Model file for the job. Use its own axes, mm. Face numbers are marked on the shaded views. Give positions to 0.01 mm unless a question says otherwise; leave off trailing zeros. Write each loop counter-clockwise with the first axis right and the second up, starting at its lowest first coordinate (ties: lowest second). Pieces come first, ordered by that corner, then holes. Notation, with made-up numbers: (71, 54) - (110, 54) arc R22 cw to (110, 63) - close; hole circle Ø7 at (18, 51). An arc over 180 degrees is marked (long way). One line per item, written item: value. Start each with the question number.
(1) Cut at C-C, the plane y = -13. List the corners of the cut face in (x, z).
(2) Probe L1, parallel to Y at x = 52.5, z = -2.5; L2, parallel to Y at x = 27, z = 11.25; L3, parallel to Y at x = 23, z = 8. List the from-to ranges inside material, lowest first.
(3) Cut at A-A, the plane z = -2.25. List the corners of the cut face in (x, y), and give its area (3 significant figures).
(4) Mould opens along X. For the marked faces 1, 2 and 3 say: pulls with the +X half, pulls with the -X half, needs draft (parallel to the pull), parting line crosses it, or undercut.
(5) Cut at D-D, the plane z = 10. State how many separate pieces and enclosed holes the cut face has, and give its area (3 significant figures).
(6) Drop flat-ended pins along their axis: P1, Ø10, axis at y = 12.5, z = 4.5, coming from the +X side; P2, Ø4.5, axis at x = 22.5, z = 9.5, coming from the -Y side; P3, Ø1, axis at y = 22, z = 3.5, coming from the -X side. Give the stop position or say it passes through.
(7) Cut at B-B, the plane y = 4. List the corners of the cut face in (x, z).
Autodesk Fusion 360 part; units mm, degrees
sketch "Sketch5" plane through (0, 0, 0) normal (1, 0, 0) x (0, 1, 0)
  line L0 (-20, 0) -> (20, 0)
  arc A0 (20, 0) -> (-20, 0) centre (0, -65.1667) ccw
  line L1 (-9.145, 3) -> (16.9339, 3) construction
  line L2 (-20, 0) -> (20, 0)
  line L3 (20, 0) -> (20, -3)
  line L4 (20, -3) -> (-20, -3)
  line L5 (-20, -3) -> (-20, 0)
  dimension "d18" = 3
  dimension "d19" = 40
  dimension "d20" = 3
extrude "Extrude5" add sketch "Sketch5" along normal blind 70 makes body 1
sketch "Sketch6" plane through (0, 0, -3) normal (0, 0, -1) x (1, 0, 0)
  line L0 (0, 20) -> (0, -20)
  line L1 (0, -20) -> (70, -20)
  line L2 (70, -20) -> (70, 20)
  line L3 (70, 20) -> (0, 20)
  line L4 (32.5, -5) -> (47.5, -5)
  arc A0 (47.5, -5) -> (47.5, 5) centre (47.5, 0) ccw
  line L5 (47.5, 5) -> (32.5, 5)
  arc A1 (32.5, 5) -> (32.5, -5) centre (32.5, 0) ccw
  line L6 (32.5, 0) -> (47.5, 0) construction
  line L7 (0, 0) -> (70, 0) construction
  line L8 (40, 5) -> (40, -5) construction
  dimension "d23" = 10
  dimension "d24" = 15
  dimension "d25" = 40
extrude "Extrude6" cut sketch "Sketch6" against normal through all contours L4 A0 L5 A1 bodies 1
ref_plane "WorkPlane3" through (0, 12.125, 0) normal (-0.9659, 0, 0.2588) x (0, 1, 0)
sketch "Sketch7" plane through (0, 12.125, 0) normal (-0.9659, 0, 0.2588) x (0, 1, 0)
  line L0 (10.375, 0) -> (-34.625, 0)
  line L1 (-34.625, 0) -> (-34.625, -25)
  line L2 (-34.625, -25) -> (10.375, -25)
  line L3 (10.375, -25) -> (10.375, 0)
  line L4 (-10.375, 0) -> (10.375, 0)
  point P0 (-12.125, 0)
  dimension "d28" = 45
  dimension "d29" = 25
extrude "Extrude7" add sketch "Sketch7" along normal blind 45 bodies 1
extrude "Extrude8" add 1 faces at (-28.9778, -6.6667, 7.7646) along direction (-0.258819, 0, -0.965926) blind 55 on bodies 1 bodies 1
ref_plane "WorkPlane4" through (16.4027, 0, 3) normal (0, 0, 1) x (0, 1, 0)
sketch "Sketch8" plane through (16.4027, 0, 3) normal (0, 0, 1) x (1, 0, 0)
  line L0 (16.0973, 5) -> (31.0973, 5)
  spline S0 degree 3 poles (31.0973, 5) (31.7254, 5) (32.3951, 4.8744) (33.627, 4.3641) (34.189, 3.9793) (35.0767, 3.0917) (35.4614, 2.5296) (35.9718, 1.2978) (36.0973, 0.6281) (36.0973, -0.6281) (35.9718, -1.2978) (35.4614, -2.5296) (35.0767, -3.0917) (34.189, -3.9793) (33.627, -4.3641) (32.3951, -4.8744) (31.7254, -5) (31.0973, -5) knots -1.507328 -1.507328 -1.507328 -1.507328 -1.318912 -1.318912 -1.130496 -1.130496 -0.94208 -0.94208 -0.753664 -0.753664 -0.565248 -0.565248 -0.376832 -0.376832 -0.188416 -0.188416 0 0 0 0
  line L1 (31.0973, -5) -> (16.0973, -5)
  spline S1 degree 3 poles (16.0973, -5) (15.4693, -5) (14.7995, -4.8744) (13.5677, -4.3641) (13.0056, -3.9793) (12.118, -3.0917) (11.7332, -2.5296) (11.2229, -1.2978) (11.0973, -0.6281) (11.0973, 0.6281) (11.2229, 1.2978) (11.7332, 2.5296) (12.118, 3.0917) (13.0056, 3.9793) (13.5677, 4.3641) (14.7995, 4.8744) (15.4693, 5) (16.0973, 5) knots 0 0 0 0 0.188416 0.188416 0.376832 0.376832 0.565248 0.565248 0.753664 0.753664 0.94208 0.94208 1.130496 1.130496 1.318912 1.318912 1.507328 1.507328 1.507328 1.507328
  line L2 (23.5973, 5) -> (23.5973, -5) construction
  circle A0 centre (23.5973, 0) radius 16
  circle A1 centre (23.5973, 0) radius 13
  dimension "d35" = 32
  dimension "d36" = 26
ref_plane "WorkPlane5" through (40, 0, 3) normal (0.2588, 0, 0.9659) x (0, -1, 0)
ref_plane "WorkPlane6" through (42.0706, 0, 10.7274) normal (0.2588, 0, 0.9659) x (0, -1, 0)
sketch "Sketch10" plane through (42.0706, 0, 10.7274) normal (0.2588, 0, 0.9659) x (0, -1, 0)
  line L0 (21, -21) -> (-21, 21) construction
  line L1 (21, -21) -> (-21, -21)
  line L2 (-21, -21) -> (-21, 21)
  line L3 (-21, 21) -> (21, 21)
  line L4 (21, 21) -> (21, -21)
  line L5 (21, -17) -> (17, -21)
  line L6 (-17, -21) -> (-21, -17)
  line L7 (-21, 17) -> (-17, 21)
  line L8 (21, 17) -> (17, 21)
  line L9 (-21, -17) -> (-23, -17)
  line L10 (-23, -17) -> (-23, 17)
  line L11 (-23, 17) -> (-21, 17)
  line L12 (-21, 17) -> (-21, -17)
  line L13 (21, -17) -> (23, -17)
  line L14 (23, -17) -> (23, 17)
  line L15 (23, 17) -> (21, 17)
  line L16 (21, 17) -> (21, -17)
  circle A0 centre (0, 0) radius 11.5
  line L17 (15.5, -15.5) -> (-15.5, -15.5) construction
  line L18 (-15.5, -15.5) -> (-15.5, 15.5) construction
  line L19 (-15.5, 15.5) -> (15.5, 15.5) construction
  line L20 (15.5, 15.5) -> (15.5, -15.5) construction
  line L21 (0, -21) -> (0, -15.5) construction
  line L22 (0, 15.5) -> (0, 21) construction
  circle A1 centre (15.5, -15.5) radius 1.75
  circle A2 centre (-15.5, -15.5) radius 1.75
  circle A3 centre (15.5, 15.5) radius 1.75
  circle A4 centre (-15.5, 15.5) radius 1.75
  circle A5 centre (15.5, -15.5) radius 3.25
  circle A6 centre (-15.5, -15.5) radius 3.25
  circle A7 centre (-15.5, 15.5) radius 3.25
  circle A8 centre (15.5, 15.5) radius 3.25
  dimension "d64" = 42
  dimension "d65" = 4
  dimension "d66" = 2
  dimension "d67" = 2
  dimension "d75" = 23
  dimension "d76" = 31
  dimension "d77" = 3.5
  dimension "d78" = 6.5
extrude "Extrude16" add sketch "Sketch10" along normal up to surface from surface at 2 separate body contours L1 L2 L3 L4 L5 L6 L7 L8 L12 L16 | A5 | A6 | A7 | A8 end surface at (34.1667, -15.0749, 1.3122) on bodies 1 makes body 2
sketch "Sketch13" plane through (0, 0, -3) normal (0, 0, -1) x (1, 0, 0)
  line L0 (32.5, 5) -> (47.5, 5)
  arc A0 (47.5, -5) -> (47.5, 5) centre (47.5, 0) ccw
  line L1 (47.5, -5) -> (32.5, -5)
  arc A1 (32.5, 5) -> (32.5, -5) centre (32.5, 0) ccw
  line L2 (0, 20) -> (0, -20)
  line L3 (0, -20) -> (70, -20)
  line L4 (70, -20) -> (70, 20)
  line L5 (70, 20) -> (0, 20)
  line L6 (25.6498, 23) -> (58.4913, 23)
  line L7 (25.6498, 21) -> (25.6498, 23)
  line L8 (58.4913, 23) -> (58.4913, 21)
  line L9 (58.4913, -21) -> (25.6498, -21)
  line L10 (58.4913, -23) -> (58.4913, -21)
  line L11 (25.6498, -23) -> (58.4913, -23)
  line L12 (21.7861, -21) -> (62.355, -21)
  line L13 (25.6498, -21) -> (25.6498, -23)
  line L14 (58.4913, 21) -> (25.6498, 21)
extrude "Extrude17" add sketch "Sketch13" along normal up to surface and the other way blind -6 contours L6 L7 L8 L14 | L9 L10 L11 L12 L13 end surface through (42.5882, 0, 12.6593) normal (0.258819, 0, 0.965926) offset 0 bodies 2
extrude "Extrude18" cut sketch "Sketch10" against normal through all from surface at -3 contours A5 | A6 | A7 | A8 bodies 2
hidden bodies 1
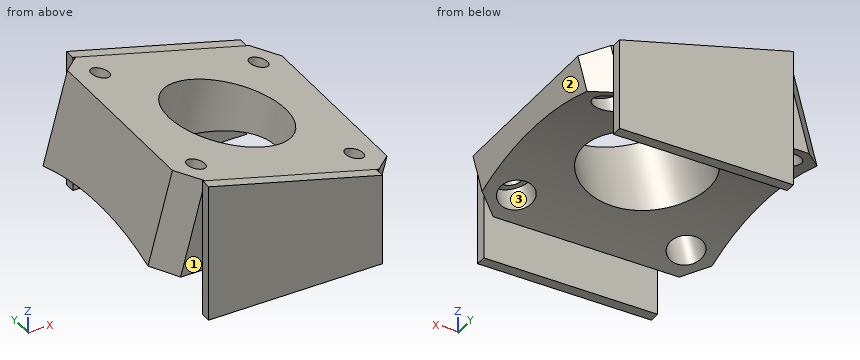
Answers follow:
1. outline: (17.92, 1.75) - (21.47, 1.75) - (24.32, 12.38) - (28.33, 11.3) - (25.77, 1.75) - (53.56, 1.75) - (54.26, 4.36) - (58.27, 3.28) - (57.86, 1.75) - (61.41, 1.75) - (62.87, 7.22) - (22.3, 18.09) - close
2. L1: y = -23 to -21, 21 to 23
2. L2: y = -23 to -18.65, -12.35 to 12.35, 18.65 to 23
2. L3: y = -20.29 to -17.88, -13.12 to 13.12, 17.88 to 20.29
3. outline: (25.65, -23) - (58.49, -23) - (58.49, -21) - (25.65, -21) - close; (25.65, 21) - (58.49, 21) - (58.49, 23) - (25.65, 23) - close
3. area: 131 mm²
4. face 1: needs draft
4. face 2: pulls with the +X half
4. face 3: undercut
5. separate pieces: 1
5. enclosed holes: 2
5. area: 961 mm²
6. P1: stops at x = 62.87
6. P2: stops at y = -21
6. P3: stops at x = 25.65
7. outline: (18.23, 2.88) - (28.81, 2.88) - (32.17, 15.45) - (22.3, 18.09) - close; (51.13, 2.88) - (61.71, 2.88) - (62.87, 7.22) - (53, 9.87) - close
